from build123d import *

# Parameters (mm, degrees)
CYLINDER052_R     = 22.5
CYLINDER052_DEPTH = 28
CYLINDER051_R     = 43
CYLINDER051_DEPTH = 28
FILLET003_R       = 2
CHAMFER001_SIZE   = 2
FILLET002_R       = 3


with BuildPart() as cylinder052:
    # Cylinder052 → Cylinder052 (new body)
    with BuildSketch(Plane.XZ):
        Circle(CYLINDER052_R)
    extrude(amount=CYLINDER052_DEPTH)


with BuildPart() as wheel_wide_right:
    # Cylinder051 → Cylinder051 (new body)
    with BuildSketch(Plane.XZ):
        Circle(CYLINDER051_R)
    extrude(amount=CYLINDER051_DEPTH)

    # Cut020: cut Cylinder052
    add(cylinder052.part, mode=Mode.SUBTRACT)

    # Fillet003
    fillet003_edges = [wheel_wide_right.edges().sort_by_distance(p)[0] for p in [
        (-43, -28, 0),
        (-43, 0, 0),
    ]]
    fillet(fillet003_edges, radius=FILLET003_R)

    # Chamfer001
    chamfer001_edges = [wheel_wide_right.edges().sort_by_distance(p)[0] for p in [
        (-22.5, 0, 0),
        (-22.5, -28, 0),
    ]]
    chamfer(chamfer001_edges, length=CHAMFER001_SIZE)

    # Fillet002
    fillet002_edges = [wheel_wide_right.edges().sort_by_distance(p)[0] for p in [
        (-24.5, 0, 0),
        (-24.5, -28, 0),
    ]]
    fillet(fillet002_edges, radius=FILLET002_R)


with BuildPart() as wheel_wide_right_1:
    # Fillet002 placement: moved
    add(wheel_wide_right.part.moved(Location((0, 91, 0))))


solid = wheel_wide_right_1.part
Work out the finished part from the listing and answer in its coordinate system (mm). Give positions to 0.01 mm unless a question says otherwise; leave off trailing zeros. Loops run counter-clockwise (first coordinate to the right, second up) from the corner with the lowest first, then second, coordinate; pieces in that order, holes last. Notation, with made-up numbers: (-31.75, 59.25) - (-25.75, 59.25) arc R11 ccw to (-25.75, 75.25) - close; hole circle Ø6 at (17, -16.5). An arc over 180 degrees is marked (long way). Answer in a Markdown table with one row per item. Add a question column.
Q1. The part is cut by section C-C (y = 81.75). Determine the outline of the cut face in (x, z), and give its area (3 significant figures).
Q2. Consider line 1 along Z through (x, y) = (0, 82.25); line 2 along Z through (x, y) = (-13.5, 77.75); line 3 along X through (y, z) = (69.25, 20.5). Determine where each line is inside the solid, lowest interval first.
Q3. Each of these flat-tipped pins is pushed along its axis until it touches: P1, Ø3, axis at x = -5.5, y = 79.5, coming from the -Z side; P2, Ø4, axis at y = 78, z = 15.5, coming from the +X side; P3, Ø2, axis at x = 0.5, z = 23.5, coming from the +Y side; P4, Ø12, axis at y = 80.5, z = -3, coming from the +X side. Where does it stop, or does it pass through?
Q4. The part is cut by section B-B (z = 0). Determine the outline of the cut face in (x, y).
Q5. Determine the mould class of faces 1 (the flat face through (-19, 63, -18)), 2 (the cylindrical face through (-5.598, 77.168, 42.634)), 3 (the cylindrical face through (10.382, 77.168, -19.961)) for opening direction Z: released by +Z, released by -Z, zero draft, split by the parting line, or undercut.
Q6. The part is cut by section A-A (x = 0). Determine the outline of the cut face in (y, z), and give its area (3 significant figures).
Solution:
| question | item | result |
|---|---|---|
| 1 | outline | circle Ø86 at (0, 0); hole circle Ø45 at (0, 0) |
| 1 | area | 4,220 mm² |
| 2 | line 1 | z = -43 to -22.5, 22.5 to 43 |
| 2 | line 2 | z = -40.83 to -18, 18 to 40.83 |
| 2 | line 3 | x = -37.8 to -9.27, 9.27 to 37.8 |
| 3 | P1 | stops at z = -42.81 |
| 3 | P2 | stops at x = 40.83 |
| 3 | P3 | stops at y = 90.73 |
| 3 | P4 | stops at x = 43 |
| 4 | outline | (-43, 65) arc R2 ccw to (-41, 63) - (-25.74, 63) arc R3 ccw to (-23.62, 63.88) - (-22.5, 65) - (-22.5, 89) - (-23.62, 90.12) arc R3 ccw to (-25.74, 91) - (-41, 91) arc R2 ccw to (-43, 89) - close; (22.5, 65) - (23.62, 63.88) arc R3 ccw to (25.74, 63) - (41, 63) arc R2 ccw to (43, 65) - (43, 89) arc R2 ccw to (41, 91) - (25.74, 91) arc R3 ccw to (23.62, 90.12) - (22.5, 89) - close |
| 5 | face 1 | zero draft |
| 5 | face 2 | split by the parting line |
| 5 | face 3 | undercut |
| 6 | outline | (63, -41) arc R2 ccw to (65, -43) - (89, -43) arc R2 ccw to (91, -41) - (91, -25.74) arc R3 ccw to (90.12, -23.62) - (89, -22.5) - (65, -22.5) - (63.88, -23.62) arc R3 ccw to (63, -25.74) - close; (63, 25.74) arc R3 ccw to (63.88, 23.62) - (65, 22.5) - (89, 22.5) - (90.12, 23.62) arc R3 ccw to (91, 25.74) - (91, 41) arc R2 ccw to (89, 43) - (65, 43) arc R2 ccw to (63, 41) - close |
| 6 | area | 1,140 mm² |
